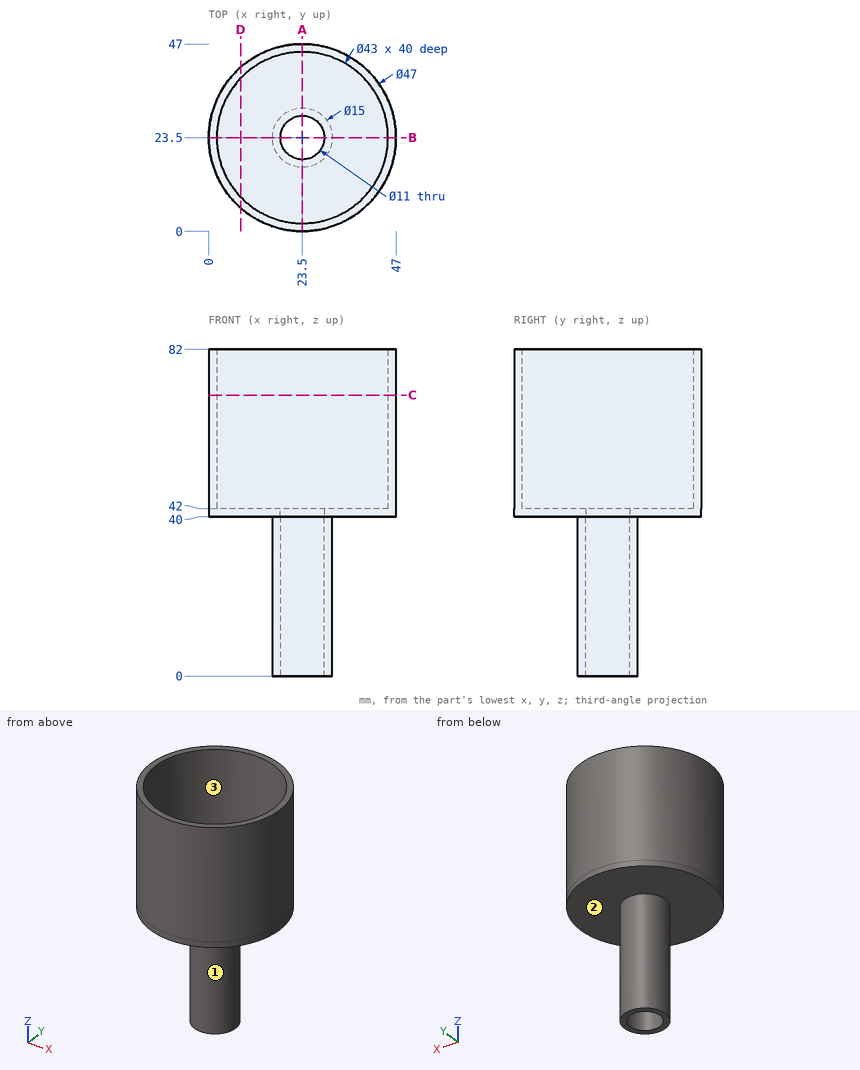
Answer from the drawing. Dimensions are ordinates in mm from the lowest x, y and z of the part. Give positions to 0.01 mm unless a question says otherwise; leave off trailing zeros. Write each loop counter-clockwise with the first axis right and the second up, starting at its lowest first coordinate (ties: lowest second). Pieces come first, ordered by that corner, then holes. Notation, with made-up numbers: (76.25, 70) -> (120.25, 70) arc R19 ccw to (120.25, 107) -> close; hole circle Ø9 at (56, -4). An arc over 180 degrees is marked (long way). Use a Markdown table: item, result.
(1) Flat-ended cylindrical pins translate along their axes: P1, Ø14.5, axis at x = 23.5, y = 23.5, coming from the -Z side; P2, Ø13, axis at x = 33, y = 32.5, coming from the +Z side; P3, Ø8, axis at x = 10.5, z = 12.5, coming from the -Y side; P4, Ø12, axis at x = 12.5, y = 32.5, coming from the -Z side. Find the tip coordinate at first contact, or state that the pin passes through.
Return value:
| item | result |
|---|---|
| P1 | z = 0 |
| P2 | z = 42 |
| P3 | through |
| P4 | z = 40 |
(2) Section A-A, the plane x = 23.5 is taken. Determine the outline of the cut face in (y, z).
Return value:
| item | result |
|---|---|
| outline | (0, 40) -> (16, 40) -> (16, 0) -> (18, 0) -> (18, 42) -> (2, 42) -> (2, 82) -> (0, 82) -> close; (29, 0) -> (31, 0) -> (31, 40) -> (47, 40) -> (47, 82) -> (45, 82) -> (45, 42) -> (29, 42) -> close |
(3) Section C-C, the plane z = 70.5 is taken. Determine the outline of the cut face in (x, y), then the cut area to 3 significant figures.
Return value:
| item | result |
|---|---|
| outline | circle Ø47 at (23.5, 23.5); hole circle Ø43 at (23.5, 23.5) |
| area | 283 mm2 |
(4) Section D-D, the plane x = 8 is taken. Determine the outline of the cut face in (y, z).
Return value:
| item | result |
|---|---|
| outline | (5.84, 40) -> (41.16, 40) -> (41.16, 82) -> (38.4, 82) -> (38.4, 42) -> (8.6, 42) -> (8.6, 82) -> (5.84, 82) -> close |
(5) Determine the mould class of the marked faces 1, 2 and 3 for opening direction Y: released by +Y, released by -Y, zero draft, split by the parting line, or undercut.
Return value:
| item | result |
|---|---|
| face 1 | split by the parting line |
| face 2 | zero draft |
| face 3 | undercut |
(6) Find the intervals of material crossed by probe 1 along Y at (x, z) = (23.5, 69); probe 2 along Z at (x, y) = (43.5, 14); probe 3 along Z at (x, y) = (17, 9.5), in increasing order. Write a range as from..to.
Return value:
| item | result |
|---|---|
| probe 1 | 0..2, 45..47 |
| probe 2 | 40..82 |
| probe 3 | 40..42 |
